```python
from build123d import *

# Parameters (mm, degrees)
SKETCH1_R             = 19.05
BOSS_EXTRUDE1_DEPTH   = 150
CUT_EXTRUDE1_DEPTH    = 153.400147638
FILLET1_R             = 3
CUT_EXTRUDE2_DEPTH    = 153.400147638
CHAMFER1_SIZE         = 1.5
F_8_0MM_DOWEL_HOLE1_D = 8
CUT_EXTRUDE3_REACH    = 157.208
SKETCH6_R             = 6


with BuildPart() as part:
    # Sketch1 → Boss-Extrude1 (new body)
    with BuildSketch(Plane(origin=(0, 0, 0), x_dir=(1, 0, 0), z_dir=(0, 1, 0))):
        with Locations(Location((0, 0, 0), (0, 0, 270))):
            Circle(SKETCH1_R)
    extrude(amount=BOSS_EXTRUDE1_DEPTH)

    # Sketch2 → Cut-Extrude1 (cut, through all)
    with BuildSketch(Plane(origin=(0, 150, 0), x_dir=(1, 0, 0), z_dir=(0, 1, 0))):
        Polygon((-11.43, -7.62), (11.43, -7.62), (11.43, 7.62), (8.89, 7.62), (8.89, -5.08), (-8.89, -5.08), (-8.89, 7.62), (-11.43, 7.62), align=None)
    extrude(amount=-CUT_EXTRUDE1_DEPTH, mode=Mode.SUBTRACT)

    # Fillet1
    fillet1_edges = [part.edges().sort_by_distance(p)[0] for p in [
        (-8.89, 75, 5.08),
        (8.89, 75, 5.08),
    ]]
    fillet(fillet1_edges, radius=FILLET1_R)

    # Sketch3 → Cut-Extrude2 (cut, through all)
    with BuildSketch(Plane(origin=(0, 150, 0), x_dir=(1, 0, 0), z_dir=(0, 1, 0))):
        with BuildLine():
            Line((-7.5, 17.511496224), (7.5, 17.511496224))
            ThreePointArc((7.5, 17.511496224), (0, 19.05), (-7.5, 17.511496224))
        make_face()
        with BuildLine():
            Line((-7.5, -17.511496224), (7.5, -17.511496224))
            ThreePointArc((7.5, -17.511496224), (0, -19.05), (-7.5, -17.511496224))
        make_face()
    extrude(amount=-CUT_EXTRUDE2_DEPTH, mode=Mode.SUBTRACT)

    # Chamfer1
    chamfer1_edges = [part.edges().sort_by_distance(p)[0] for p in [
        (19.05, 0, 0),
        (-19.05, 0, 0),
        (-19.05, 150, 0),
        (19.05, 150, 0),
    ]]
    chamfer(chamfer1_edges, length=CHAMFER1_SIZE)

    # Ø8.0mm Dowel Hole1 (through all)
    with Locations(Plane(origin=(0, 0, -17.511496224), x_dir=(-1, 0, 0), z_dir=(0, 0, -1))):
        with Locations((0, 130), (0, 75), (0, 20)):
            Hole(F_8_0MM_DOWEL_HOLE1_D / 2)

    # Cut-Extrude3: up to this face of the body (flat: up to its plane)
    cut_extrude3_end = Plane(part.part.faces().sort_by_distance((0, 148.482680666, 7.62))[0])
    # Sketch6 → Cut-Extrude3 (cut, up to the picked face)
    with BuildSketch(Plane(origin=(0, 0, -17.511496224), x_dir=(-1, 0, 0), z_dir=(0, 0, -1)), mode=Mode.PRIVATE) as cut_extrude3_sk1:
        with Locations((0, 130)):
            Circle(SKETCH6_R)
    cut_extrude3_tool1 = split(extrude(cut_extrude3_sk1.sketch, amount=-CUT_EXTRUDE3_REACH, mode=Mode.PRIVATE), bisect_by=cut_extrude3_end, keep=Keep.BOTH, mode=Mode.PRIVATE)
    # Sketch6 → Cut-Extrude3 (cut, up to the picked face)
    with BuildSketch(Plane(origin=(0, 0, -17.511496224), x_dir=(-1, 0, 0), z_dir=(0, 0, -1)), mode=Mode.PRIVATE) as cut_extrude3_sk2:
        with Locations((0, 75)):
            Circle(SKETCH6_R)
    cut_extrude3_tool2 = split(extrude(cut_extrude3_sk2.sketch, amount=-CUT_EXTRUDE3_REACH, mode=Mode.PRIVATE), bisect_by=cut_extrude3_end, keep=Keep.BOTH, mode=Mode.PRIVATE)
    # Sketch6 → Cut-Extrude3 (cut, up to the picked face)
    with BuildSketch(Plane(origin=(0, 0, -17.511496224), x_dir=(-1, 0, 0), z_dir=(0, 0, -1)), mode=Mode.PRIVATE) as cut_extrude3_sk3:
        with Locations((0, 20)):
            Circle(SKETCH6_R)
    cut_extrude3_tool3 = split(extrude(cut_extrude3_sk3.sketch, amount=-CUT_EXTRUDE3_REACH, mode=Mode.PRIVATE), bisect_by=cut_extrude3_end, keep=Keep.BOTH, mode=Mode.PRIVATE)
    add(cut_extrude3_tool1.solids().sort_by(Axis((0, 130, -17.511496), (0, 0, 1)))[0], mode=Mode.SUBTRACT)
    add(cut_extrude3_tool2.solids().sort_by(Axis((0, 75, -17.511496), (0, 0, 1)))[0], mode=Mode.SUBTRACT)
    add(cut_extrude3_tool3.solids().sort_by(Axis((0, 20, -17.511496), (0, 0, 1)))[0], mode=Mode.SUBTRACT)


solid = part.part
```
CAD build for the part. Positions are in the model's coordinates, mm. A direction names the side the tool comes from. Coordinates: 2 decimals unless noted, no trailing zeros. Order: outer loops, then holes, each group sorted by start corner. A loop starts at its lowest first (then second) coordinate and runs counter-clockwise, first axis right, second up. Notation, with made-up numbers: (11.25, -23) - (33.25, -23) arc R27 ccw to (33.25, 10) - close; hole circle Ø2 at (9.25, -25.5). An arc over 180 degrees is marked (long way). Answer in a Markdown table with one row per item.
1. Pull direction Y, two halves, no side cores. Call faces 4 (the face through (-17.786, 149.76, -0.375)), 5 (the face through (2.15, 133.373, 12.635)), 6 (the face through (5, 76, 7.62)): +Y half, -Y half, draft (parallel to the pull), parting line (faces both ways), or undercut.
Answer:
| item | result |
|---|---|
| face 4 | +Y half |
| face 5 | undercut |
| face 6 | draft |
2. Drill centre lines: L1, parallel to Y at x = 0, z = -3.5; L2, parallel to Y at x = 0, z = 14.25; L3, parallel to Z at x = -5, y = 42. Where is each one in solid material? Low to high. Write a range as from..to.
Answer:
| item | result |
|---|---|
| L1 | 0..14, 26..69, 81..124, 136..150 |
| L2 | 0..16, 24..71, 79..126, 134..150 |
| L3 | -17.51..5.08, 7.62..17.51 |
3. Slice it at C-C, the plane z = -11. Give the number of separate pieces and of enclosed holes in the cut face, then the cut area to 3 significant figures.
Answer:
| item | result |
|---|---|
| separate pieces | 1 |
| enclosed holes | 3 |
| area | 4,320 mm² |
4. Slice it at A-A, the plane z = 0. List the corners of the cut face in (x, y).
Answer:
| item | result |
|---|---|
| outline | (-19.05, 1.5) - (-17.55, 0) - (-11.43, 0) - (-11.43, 150) - (-17.55, 150) - (-19.05, 148.5) - close; (-8.89, 0) - (8.89, 0) - (8.89, 150) - (-8.89, 150) - close; (11.43, 0) - (17.55, 0) - (19.05, 1.5) - (19.05, 148.5) - (17.55, 150) - (11.43, 150) - close; hole circle Ø12 at (0, 20); hole circle Ø12 at (0, 75); hole circle Ø12 at (0, 130) |
5. Flat gauge pins, fed straight in: P1, Ø15.5, axis at x = 0, y = 20, coming from the -Z side; P2, Ø3, axis at y = 90, z = -10, coming from the +X side; P3, Ø0.8, axis at x = -10.5, y = 62, coming from the +Z side; P4, Ø5, axis at x = 0, y = 130, coming from the -Z side. Where does each tip first touch, or does it go through?
Answer:
| item | result |
|---|---|
| P1 | z = -17.51 |
| P2 | x = 17.05 |
| P3 | z = 16.15 |
| P4 | through |
6. Slice it at B-B, the plane y = 62.5. List the corners of the cut face in (x, z), then the cut area to 3 significant figures.
Answer:
| item | result |
|---|---|
| outline | (-7.5, -17.51) - (7.5, -17.51) arc R19.05 ccw to (7.5, 17.51) - (-7.5, 17.51) arc R19.05 ccw to start; hole (-11.43, -7.62) - (-8.89, -7.62) - (-8.89, 2.08) arc R3 cw to (-5.89, 5.08) - (5.89, 5.08) arc R3 cw to (8.89, 2.08) - (8.89, -7.62) - (11.43, -7.62) - (11.43, 7.62) - (-11.43, 7.62) - close |
| area | 983 mm² |
7. 3-axis set-ups, long thin cutter, end or side, ignore diameter. For faces 1 (the face through (0.78, 80.95, -6.37)), 2 (the face through (-0.521, 23.966, 12.635)), 3 (the face through (0, 143, 5.08)): which of +Z, -Z, +X, -X, +Y, -Y reach the whole face in a straight line?
Answer:
| item | result |
|---|---|
| face 1 | -Z |
| face 2 | +Z, -Z |
| face 3 | +Y, -Y |
